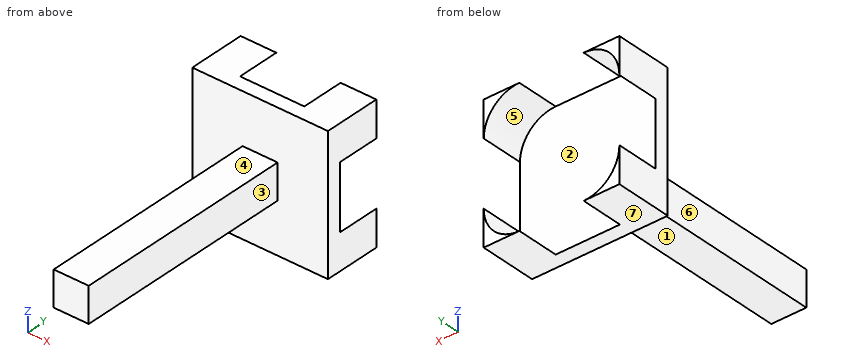
Autodesk Inventor part; units mm, degrees
ref_plane "YZ Plane" through (0, 0, 0) normal (1, 0, 0) x (0, 1, 0)
ref_plane "XZ Plane" through (0, 0, 0) normal (0, 1, 0) x (-1, 0, 0)
ref_plane "XY Plane" through (0, 0, 0) normal (0, 0, 1) x (1, 0, 0)
sketch "Sketch1" plane through (0, 0, 0) normal (0, 1, 0) x (-1, 0, 0)
  line L0 (-9.5, 9.5) -> (9.5, 9.5)
  line L1 (9.5, 9.5) -> (9.5, -9.5)
  line L2 (9.5, -9.5) -> (-9.5, -9.5)
  line L3 (-9.5, -9.5) -> (-9.5, 9.5)
  line L4 (-9.5, 9.5) -> (9.5, -9.5) construction
  line L5 (9.5, 9.5) -> (-9.5, -9.5) construction
  line L6 (9.5, 0) -> (9.5, 4.5)
  line L7 (9.5, 0) -> (14, 0) construction
  line L8 (0, 9.5) -> (4.5, 9.5)
  line L9 (0, 9.5) -> (4.5, 9.5) construction
  arc A0 (9.5, 4.5) -> (4.5, 9.5) centre (4.5, 4.5) ccw
  arc A1 (-4.5, 9.5) -> (-9.5, 4.5) centre (-4.5, 4.5) ccw
  arc A2 (-9.5, -4.5) -> (-4.5, -9.5) centre (-4.5, -4.5) ccw
  arc A3 (4.5, -9.5) -> (9.5, -4.5) centre (4.5, -4.5) ccw
  point P0 (0, 0)
  point P1 (9.5, -4.5)
  point P2 (-4.5, 9.5)
  point P3 (-9.5, 4.5)
  point P4 (-9.5, -4.5)
  point P5 (-4.5, -9.5)
  dimension "d0" = 19
  dimension "d1" = 19
  dimension "d2" = 4.5
  dimension "d3" = 90
  dimension "d4" = 4.5
  dimension "d5" = 0
  dimension "d6" = 5
  dimension "d9" = 360
extrude "Extrusion1" add sketch "Sketch1" along normal blind 2 contours L0 A0 L1 A3 L2 A2 L3 A1
extrude "Extrusion2" add sketch "Sketch1" along normal blind 8 contours L0 A1 L3 | A2 L2 L3 | L0 L1 A0 | A3 L1 L2
sketch "Sketch2" plane through (0, 0, 0) normal (0, -1, 0) x (1, 0, 0)
  line L0 (-2.45, 2.45) -> (-2.45, -2.45)
  line L1 (-2.45, -2.45) -> (2.45, -2.45)
  line L2 (2.45, -2.45) -> (2.45, 2.45)
  line L3 (2.45, 2.45) -> (-2.45, 2.45)
  line L4 (-2.45, 2.45) -> (2.45, -2.45) construction
  line L5 (-2.45, -2.45) -> (2.45, 2.45) construction
  line L6 (-2.45, 2.45) -> (2.45, 2.45) construction
  point P0 (0, 0)
  dimension "d22" = 4.9
  dimension "d23" = 90
  dimension "d24" = 4.9
extrude "Extrusion3" add sketch "Sketch2" along normal blind 31.25
properties part number "CenterClawv2.2"
Build history of the part. All positions in model axes, mm. Face numbers are marked on the shaded views. A direction names the side the tool comes from. Coordinates: 2 decimals unless noted, no trailing zeros. Order: outer loops, then holes, each group sorted by start corner. A loop starts at its lowest first (then second) coordinate and runs counter-clockwise, first axis right, second up. Notation, with made-up numbers: (83, 61) -> (111, 61) arc R16 cw to (111, 76) -> close; hole circle Ø7 at (71.25, 20.25). An arc over 180 degrees is marked (long way). Answer in a Markdown table with one row per item. Add a question column.
Q1. Wall check: line 1 along Y through (x, z) = (7.25, -5.5); line 2 along Z through (x, y) = (-1.25, -20); line 3 along Z through (x, y) = (7, 3). Give the ranges that are in metal, low to high. Write a range as [from, to].
Q2. Mould opens along X. For the marked faces 5, 6 and 7 say: +X half, -X half, draft (parallel to the pull), parting line (faces both ways), or undercut.
Q3. Band-saw the part on B-B, the plane x = 0. List the corners of the cut face in (y, z).
Q4. Which spindle directions (+Z, -Z, +X, -X, +Y, -Y) get a long thin tool onto all of the face, cutting with end or side? Do the marked faces 1, 2, 3 and 4. Say none if no direction does.
Q5. Band-saw the part on D-D, the plane x = -3.5. List the corners of the cut face in (y, z), then the cut area to 3 significant figures.
Q6. Band-saw the part on A-A, the plane z = 1.5. List the corners of the cut face in (x, y).
Q7. Band-saw the part on C-C, the plane y = -27. List the corners of the cut face in (x, z), then the cut area to 3 significant figures.
Q8. Drop flat-ended pins along their axis: pin 1 (8 mm diameter, centred on x = 0.5, y = -14.5, fed in from +Z); pin 2 (5.5 mm diameter, centred on x = 1, y = -15.5, fed in from -Z); pin 3 (1.5 mm diameter, centred on x = 4, z = -2.5, fed in from -Y). Give the stop position or say it passes through.
Answers follow:
| question | item | result |
|---|---|---|
| 1 | line 1 | [0, 2] |
| 1 | line 2 | [-2.45, 2.45] |
| 1 | line 3 | [-9.5, -8.83], [8.83, 9.5] |
| 2 | face 5 | undercut |
| 2 | face 6 | -X half |
| 2 | face 7 | draft |
| 3 | outline | (-31.25, -2.45) -> (0, -2.45) -> (0, -9.5) -> (2, -9.5) -> (2, 9.5) -> (0, 9.5) -> (0, 2.45) -> (-31.25, 2.45) -> close |
| 4 | face 1 | -Z, +X, -X, -Y |
| 4 | face 2 | +Y |
| 4 | face 3 | +Z, -Z, +X, -Y |
| 4 | face 4 | +Z, +X, -X, -Y |
| 5 | outline | (0, -9.5) -> (2, -9.5) -> (2, 9.5) -> (0, 9.5) -> close |
| 5 | area | 38.0 mm^2 |
| 6 | outline | (-9.5, 0) -> (-2.45, 0) -> (-2.45, -31.25) -> (2.45, -31.25) -> (2.45, 0) -> (9.5, 0) -> (9.5, 2) -> (-9.5, 2) -> close |
| 7 | outline | (-2.45, -2.45) -> (2.45, -2.45) -> (2.45, 2.45) -> (-2.45, 2.45) -> close |
| 7 | area | 24.0 mm^2 |
| 8 | pin 1 | z = 2.45 |
| 8 | pin 2 | z = -2.45 |
| 8 | pin 3 | y = 0 |
